Input: dimensioned drawing with shaded views. Units: mm. Origin: part minimum x, y, z. A direction names the side the tool comes from. Round coordinates to 2 decimals unless told otherwise and drop trailing zeros. Order: outer loops, then holes, each group sorted by start corner. A loop starts at its lowest first (then second) coordinate and runs counter-clockwise, first axis right, second up. Notation, with made-up numbers: M -2,23 L 55,23 A25 ccw 55,36 Z; hole C -13.5,-13 d5. An arc over 180 degrees is marked long. One line per question, with ' | ' between items.
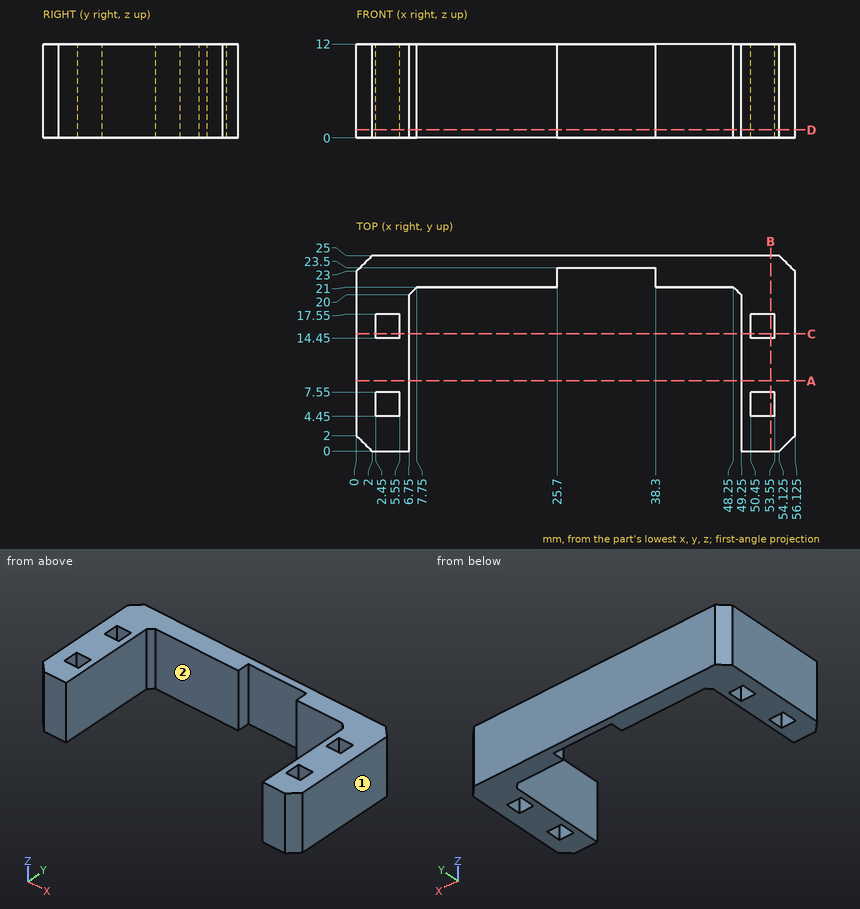
Item 1: Line query: line 1 along X through (y, z) = (7.5, 11.75) (3 decimals); line 2 along Y through (x, z) = (52, 4.5); line 3 along X through (y, z) = (8.25, 3.75) (3 decimals). Output: solid intervals per line, ascending. Write a range as from..to.
Report:
line 1: 0..2.45, 5.55..6.75, 49.25..50.45, 53.55..56.125 | line 2: 0..4.45, 7.55..14.45, 17.55..25 | line 3: 0..6.75, 49.25..56.125
Item 2: Section query C-C, the plane y = 15. Return loops of the section in (x, z) (3 decimals), plus the area to 3 significant figures.
Report:
outline: M 0,0 L 2.45,0 L 2.45,12 L 0,12 Z; M 5.55,0 L 6.75,0 L 6.75,12 L 5.55,12 Z; M 49.25,0 L 50.45,0 L 50.45,12 L 49.25,12 Z; M 53.55,0 L 56.125,0 L 56.125,12 L 53.55,12 Z | area: 89.1 mm²
Item 3: First-contact query: pin 1 (5 mm diameter, centred on x = 44.5, z = 8.5, fed in from -Y); pin 2 (1.5 mm diameter, centred on x = 8, y = 13.5, fed in from +Z); pin 3 (6 mm diameter, centred on x = 33, z = 7.5, fed in from -Y). Flat tips, straight axial feed; report the tip coordinate or a pass-through.
Report:
pin 1: y = 21 | pin 2: through | pin 3: y = 23.5
Item 4: Section query A-A, the plane y = 9. Return loops of the section in (x, z) (3 decimals).
Report:
outline: M 0,0 L 6.75,0 L 6.75,12 L 0,12 Z; M 49.25,0 L 56.125,0 L 56.125,12 L 49.25,12 Z
Item 5: Section query D-D, the plane z = 1. Give the number of separate pieces and of enclosed holes in the cut face, plus the area to 3 significant figures.
Report:
separate pieces: 1 | enclosed holes: 4 | area: 434 mm²
Item 6: Access query for the marked faces 1 and 2. Directions: +Z, -Z, +X, -X, +Y, -Y. A direction counts if a zero-diameter tool reaches every point of the face in a straight line with its end or side. Return the directions, or none.
Report:
face 1: +Z, -Z, +X, +Y, -Y | face 2: +Z, -Z, -Y
Item 7: Section query B-B, the plane x = 53. Return loops of the section in (y, z), plus the area to 3 significant figures.
Report:
outline: M 0,0 L 4.45,0 L 4.45,12 L 0,12 Z; M 7.55,0 L 14.45,0 L 14.45,12 L 7.55,12 Z; M 17.55,0 L 25,0 L 25,12 L 17.55,12 Z | area: 226 mm²
